Part model, mm, in its own coordinate system. A direction names the side the tool comes from. Give positions to 0.01 mm unless a question says otherwise; leave off trailing zeros. Write each loop counter-clockwise with the first axis right and the second up, starting at its lowest first coordinate (ties: lowest second). Pieces come first, ordered by that corner, then holes. Notation, with made-up numbers: M -12.75,64 L 5.25,64 A21 ccw 5.25,99 Z; hole C 37,67.25 d4. An arc over 180 degrees is marked long. Answer as CSV lines item,"result". Start each with the question number.
Item 1: Band-saw the part on A-A, the plane x = 13. List the corners of the cut face in (y, z).
Item 2: Two-plate mould, pull along Y, no slides. Class faces 1 (the flat face through (12.1, -15, 1)), 2 (the flat face through (-24.5, 25, 1)), 3 (the flat face through (0, -27, 1)), 4 (the cylindrical face through (-11.06, -8.835, 0.986)): +Y half, -Y half, draft (parallel to the pull), parting line (faces both ways), or undercut.
Item 3: Pin check, flat tips, straight feed: pin 1 (1 mm diameter, centred on y = 12.5, z = 1, fed in from -X); pin 2 (1 mm diameter, centred on y = 45.5, z = 0.5, fed in from +X); pin 3 (0.6 mm diameter, centred on y = 49, z = 1, fed in from -X). Stop position of each tip, or through.
Item 4: Wall check: L1, parallel to Y at x = -24, z = 1.6; L2, parallel to X at y = 12, z = 0.8; L3, parallel to Y at x = -12, z = 1.3. Give the ranges that are in metal, low to high. Write a range as from..to.
Item 5: Band-saw the part on D-D, the plane y = 47. List the corners of the cut face in (x, z), then the cut area to 3 significant figures.
Item 6: Band-saw the part on C-C, the plane x = 0. List the corners of the cut face in (y, z), then the cut area to 3 significant figures.
Item 7: Band-saw the part on B-B, the plane y = 0. List the corners of the cut face in (x, z), then the cut area to 3 significant figures.
Item 8: 3-axis set-ups, long thin cutter, end or side, ignore diameter. For faces 5 (the flat face through (-12.1, -15, 1)), 6 (the flat face through (21, -12.95, 1)), 7 (the flat face through (0, 14, 0)), 8 (the flat face through (17, -11.5, 1)): which of +Z, -Z, +X, -X, +Y, -Y reach the whole face in a straight line?
from build123d import *

# Parameters (mm, degrees)
SKETCH_1_R          = 1.575
SKETCH_1_R_2        = 11.5
SKETCH_1_R_3        = 2
EXTRUDE_1_DEPTH     = 2
FILLET_1_R          = 1.3
SKETCH_4_W          = 3
SKETCH_4_H          = 5.878615105
SKETCH_4_H_2        = 11.344283934
CUT_EXTRUDE_1_DEPTH = 2


with BuildPart() as part:
    # 草图1 → 凸台-拉伸1 (new body)
    with BuildSketch(Plane.XY):
        Polygon((22.5, -27), (-22.5, -27), (-27.5, -27), (-27.5, -23), (-22.5, -23), (-22.5, -17.05), (-18.5, -17.05), (-18.5, -18.5), (-15.3, -18.5), (-15.3, -17.05), (-12.1, -17.05), (-12.1, -12.95), (-15.3, -12.95), (-15.3, -11.5), (-18.5, -11.5), (-18.5, -12.95), (-22.5, -12.95), (-22.5, -4), (-27.5, -4), (-27.5, 4), (-22.5, 4), (-22.5, 12.95), (-18.5, 12.95), (-18.5, 11.5), (-15.3, 11.5), (-15.3, 12.95), (-12.1, 12.95), (-12.1, 17.05), (-15.3, 17.05), (-15.3, 18.5), (-18.5, 18.5), (-18.5, 17.05), (-22.5, 17.05), (-22.5, 23), (-27.5, 23), (-27.5, 27), (-22.5, 27), (-9, 27), (-9, 41), (-22, 41), (-22, 53), (22, 53), (22, 41), (9, 41), (9, 27), (22.5, 27), (27.5, 27), (27.5, 23), (22.5, 23), (22.5, 17.05), (18.5, 17.05), (18.5, 18.5), (15.3, 18.5), (15.3, 17.05), (12.1, 17.05), (12.1, 12.95), (15.3, 12.95), (15.3, 11.5), (18.5, 11.5), (18.5, 12.95), (22.5, 12.95), (22.5, 4), (27.5, 4), (27.5, -4), (22.5, -4), (22.5, -12.95), (18.5, -12.95), (18.5, -11.5), (15.3, -11.5), (15.3, -12.95), (12.1, -12.95), (12.1, -17.05), (15.3, -17.05), (15.3, -18.5), (18.5, -18.5), (18.5, -17.05), (22.5, -17.05), (22.5, -23), (27.5, -23), (27.5, -27), align=None)
        with Locations((9.899494937, 9.899494937)):
            Circle(SKETCH_1_R, mode=Mode.SUBTRACT)
        Circle(SKETCH_1_R_2, mode=Mode.SUBTRACT)
        with Locations((9.899494937, -9.899494937)):
            Circle(SKETCH_1_R, mode=Mode.SUBTRACT)
        with Locations((-9.899494937, -9.899494937)):
            Circle(SKETCH_1_R, mode=Mode.SUBTRACT)
        with Locations((-9.899494937, 9.899494937)):
            Circle(SKETCH_1_R, mode=Mode.SUBTRACT)
        with Locations((-18, 47)):
            Circle(SKETCH_1_R_3, mode=Mode.SUBTRACT)
        with Locations((18, 47)):
            Circle(SKETCH_1_R_3, mode=Mode.SUBTRACT)
        with Locations((0, 29)):
            Circle(SKETCH_1_R_3, mode=Mode.SUBTRACT)
    extrude(amount=EXTRUDE_1_DEPTH)

    # 圆角1
    fillet_1_edges = [part.edges().sort_by_distance(p)[0] for p in [
        (-9, 27, 1),
        (-9, 41, 1),
        (-22, 41, 1),
        (-22, 53, 1),
        (22, 53, 1),
        (22, 41, 1),
        (9, 41, 1),
        (9, 27, 1),
        (27.5, 23, 1),
        (27.5, 4, 1),
        (27.5, -4, 1),
        (27.5, -23, 1),
        (-27.5, -23, 1),
        (-27.5, -4, 1),
        (-27.5, 4, 1),
        (-27.5, 23, 1),
    ]]
    fillet(fillet_1_edges, radius=FILLET_1_R)

    # 草图4 → 切除-拉伸1 (cut)
    with BuildSketch(Plane.XY.offset(2)):
        with Locations((26, 24.060692448)):
            Rectangle(SKETCH_4_W, SKETCH_4_H)
        with Locations((-26, 21.327858033)):
            Rectangle(SKETCH_4_W, SKETCH_4_H_2)
    extrude(amount=-CUT_EXTRUDE_1_DEPTH, mode=Mode.SUBTRACT)


solid = part.part
Output:
1,outline,"M -27,0 L -17.05,0 L -17.05,2 L -27,2 Z; M -12.95,0 L 12.95,0 L 12.95,2 L -12.95,2 Z; M 17.05,0 L 27,0 L 27,2 L 17.05,2 Z; M 41,0 L 53,0 L 53,2 L 41,2 Z"
2,face 1,"undercut"
2,face 2,"draft"
2,face 3,"-Y half"
2,face 4,"undercut"
3,pin 1,"x = -22.5"
3,pin 2,"x = 22"
3,pin 3,"x = -22"
4,L1,"-27..-23, -4..4, 23..27"
4,L2,"-22.5..-18.5, -15.3..15.3, 18.5..22.5"
4,L3,"-27..27, 41..53"
5,outline,"M -22,0 L -20,0 L -20,2 L -22,2 Z; M -16,0 L 16,0 L 16,2 L -16,2 Z; M 20,0 L 22,0 L 22,2 L 20,2 Z"
5,area,"72.0 mm²"
6,outline,"M -27,0 L -11.5,0 L -11.5,2 L -27,2 Z; M 11.5,0 L 27,0 L 27,2 L 11.5,2 Z; M 31,0 L 53,0 L 53,2 L 31,2 Z"
6,area,"106 mm²"
7,outline,"M -27.5,0 L -11.5,0 L -11.5,2 L -27.5,2 Z; M 11.5,0 L 27.5,0 L 27.5,2 L 11.5,2 Z"
7,area,"64.0 mm²"
8,face 5,"+Z, -Z, -X"
8,face 6,"+Z, -Z, +X"
8,face 7,"-Z, +X, -X, +Y, -Y"
8,face 8,"+Z, -Z"
